Answer from the drawing. Dimensions are ordinates in mm from the lowest x, y and z of the part. A direction names the side the tool comes from. Round coordinates to 2 decimals unless told otherwise and drop trailing zeros. Loops run counter-clockwise (first coordinate to the right, second up) from the corner with the lowest first, then second, coordinate; pieces in that order, holes last. Notation, with made-up numbers: M 68,28.5 L 121,28.5 A15 ccw 121,51.5 Z; hole C 15.25,28.5 d4. An arc over 180 degrees is marked long. Answer as CSV lines item,"result".
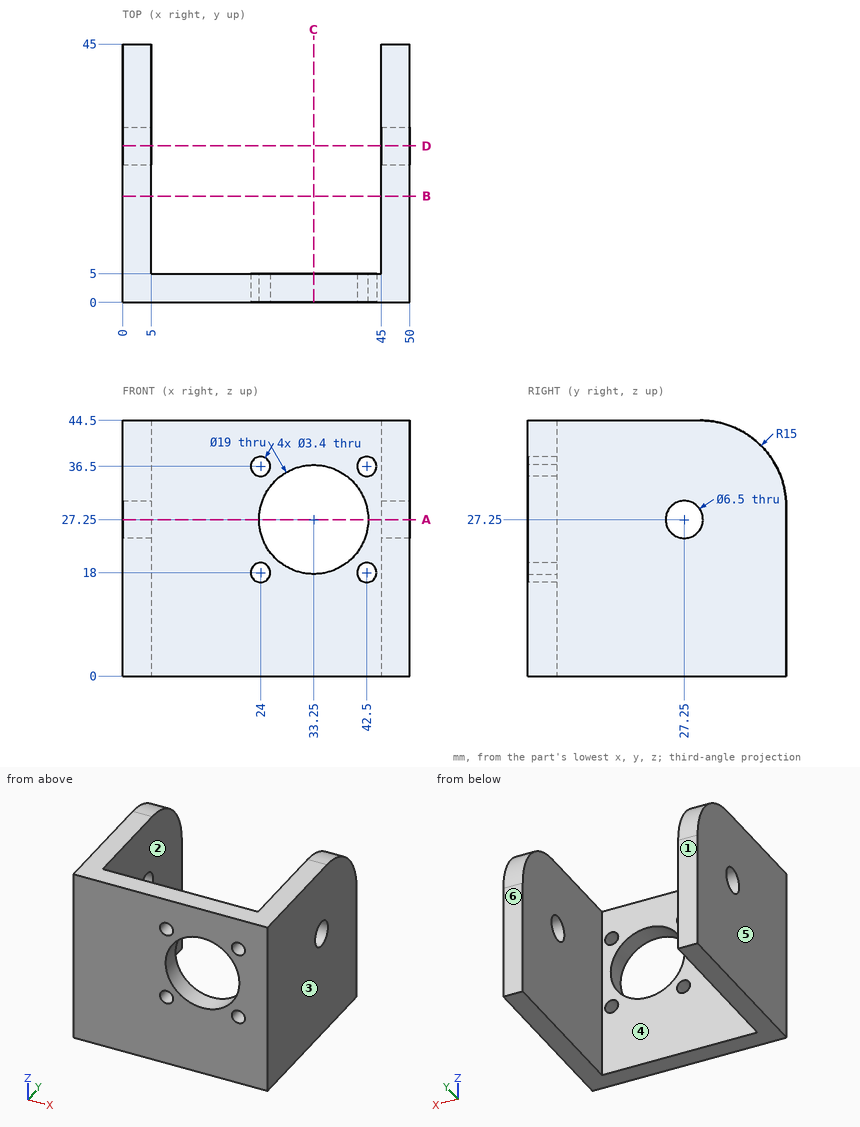
1) Find section C-C, the plane x = 33.25. Give the vertices of the cut face in (y, z).
Evaluation:
outline,"M 0,0 L 5,0 L 5,17.75 L 0,17.75 Z; M 0,36.75 L 5,36.75 L 5,44.5 L 0,44.5 Z"
2) Find section D-D, the plane y = 27.25. Give the vertices of the cut face in (x, z).
Evaluation:
outline,"M 0,0 L 5,0 L 5,24 L 0,24 Z; M 0,30.5 L 5,30.5 L 5,44.5 L 0,44.5 Z; M 45,0 L 50,0 L 50,24 L 45,24 Z; M 45,30.5 L 50,30.5 L 50,44.5 L 45,44.5 Z"
3) Find section A-A, the plane z = 27.25. Give the vertices of the cut face in (x, y), then the cut area to 3 significant figures.
Evaluation:
outline,"M 0,0 L 23.75,0 L 23.75,5 L 5,5 L 5,24 L 0,24 Z; M 0,30.5 L 5,30.5 L 5,45 L 0,45 Z; M 42.75,0 L 50,0 L 50,24 L 45,24 L 45,5 L 42.75,5 Z; M 45,30.5 L 50,30.5 L 50,45 L 45,45 Z"
area,"490 mm^2"
4) Determine the mould class of the marked faces 3, 4, 5 and 6 for opening direction X: released by +X, released by -X, zero draft, split by the parting line, or undercut.
Evaluation:
face 3,"released by +X"
face 4,"undercut"
face 5,"released by -X"
face 6,"zero draft"
5) A tool of negligible diameter and unlimited length cuts with its end or side. For the marked faces 1 and 2, from which of +Z, -Z, +X, -X, +Y, -Y can it reach the whole face along a straight path? Write none if from no direction.
Evaluation:
face 1,"+Z, -Z, +X, -X, +Y"
face 2,"+Z, -Z, +Y"
6) Each of these flat-tipped pins is pushed along its axis until it touches: P1, Ø2, axis at y = 23, z = 17.5, coming from the -X side; P2, Ø12, axis at x = 18, z = 26.5, coming from the +Y side. Where does it stop, or does it pass through?
Evaluation:
P1,"stops at x = 0"
P2,"stops at y = 5"
7) Straight lines are drawn through the part: line 1 (X direction, y = 14, z = 23); line 2 (X direction, y = 3, z = 36); line 3 (Z direction, x = 48, y = 27). For each, find the intervals that lie inside material, in ascending order.
Evaluation:
line 1,"x = 0 to 5, 45 to 50"
line 2,"x = 0 to 22.38, 25.62 to 29.55, 36.95 to 40.88, 44.12 to 50"
line 3,"z = 0 to 24.01, 30.49 to 44.5"
8) Find section B-B, the plane y = 18.5. Give the vertices of the cut face in (x, z).
Evaluation:
outline,"M 0,0 L 5,0 L 5,44.5 L 0,44.5 Z; M 45,0 L 50,0 L 50,44.5 L 45,44.5 Z"
